from build123d import *

# Parameters (mm, degrees)
SKETCH2_W           = 500
SKETCH2_H           = 500
BOSS_EXTRUDE1_DEPTH = 50
SKETCH7_W           = 400
SKETCH7_H           = 400
CUT_EXTRUDE1_DEPTH  = 550
SKETCH8_W           = 500
SKETCH8_H           = 10
BOSS_EXTRUDE2_DEPTH = 10
SKETCH9_W           = 50
SKETCH9_H           = 50
BOSS_EXTRUDE3_DEPTH = 550
SKETCH10_W          = 50
SKETCH10_H          = 50
BOSS_EXTRUDE4_DEPTH = 600


with BuildPart() as part:
    # Sketch2 → Boss-Extrude1 (new body)
    with BuildSketch(Plane(origin=(0, 0, 0), x_dir=(1, 0, 0), z_dir=(0, 1, 0))):
        Rectangle(SKETCH2_W, SKETCH2_H)
    extrude(amount=BOSS_EXTRUDE1_DEPTH)

    # Sketch7 → Cut-Extrude1 (cut)
    with BuildSketch(Plane(origin=(0, 50, 0), x_dir=(1, 0, 0), z_dir=(0, 1, 0))):
        Rectangle(SKETCH7_W, SKETCH7_H)
    extrude(amount=-CUT_EXTRUDE1_DEPTH, mode=Mode.SUBTRACT)

    # Sketch8 → Boss-Extrude2 (add)
    with BuildSketch(Plane(origin=(0, 50, 0), x_dir=(1, 0, 0), z_dir=(0, 1, 0))):
        with Locations((0, 235)):
            Rectangle(SKETCH8_W, SKETCH8_H)
        with Locations((0, -235)):
            Rectangle(SKETCH8_W, SKETCH8_H)
    extrude(amount=BOSS_EXTRUDE2_DEPTH)

    # Sketch9 → Boss-Extrude3 (add)
    with BuildSketch(Plane.XZ):
        with Locations((125, -275)):
            Rectangle(SKETCH9_W, SKETCH9_H)
        with Locations((125, 275)):
            Rectangle(SKETCH9_W, SKETCH9_H)
    extrude(amount=-BOSS_EXTRUDE3_DEPTH)

    # Sketch10 → Boss-Extrude4 (add)
    with BuildSketch(Plane.XY.offset(300)):
        with Locations((125, 575)):
            Rectangle(SKETCH10_W, SKETCH10_H)
    extrude(amount=-BOSS_EXTRUDE4_DEPTH)


solid = part.part
Check sheet for the modelled part. Datum: model origin and axes. Units: mm. A direction names the side the tool comes from. Give positions to 0.01 mm unless a question says otherwise; leave off trailing zeros. Loops run counter-clockwise (first coordinate to the right, second up) from the corner with the lowest first, then second, coordinate; pieces in that order, holes last. Notation, with made-up numbers: M 45.5,-12 L 65.5,-12 A5 cw 65.5,-6 Z; hole C -20,35 d4. An arc over 180 degrees is marked long. Use a Markdown table: item, result. Add a question column.
Q1. Sectioned sample at C-C, the plane z = 178.5. Record the cut outline in (x, y).
Q2. Sectioned sample at D-D, the plane x = -217.5. Record the cut outline in (y, z), then the cut area to 3 significant figures.
Q3. Scan lines: line 1 along Y through (x, z) = (24, 244); line 2 along X through (y, z) = (430.5, 250.5); line 3 along Z through (x, y) = (-93, 42). Record each from-to range of solid material in increasing order. Write a range as [from, to].
Q4. Sectioned sample at B-B, the plane x = -18. Record the cut outline in (y, z), then the cut area to 3 significant figures.
Q5. Mould release check, pull along Y, two halves, no side actions. Record for faces 1 (the flat face through (125, 296, -250)), 2 (the flat face through (200, 25, 3)), 3 (the flat face through (125, 600, 4)): pulls with the +Y half, pulls with the -Y half, needs draft (parallel to the pull), parting line crosses it, or undercut.
Q6. Tool access check on faces 4 (the flat face through (199, 25, 250)), 5 (the flat face through (-200, 25, 3)), 6 (the flat face through (-77, 25, 250)). Record the directions out of +Z, -Z, +X, -X, +Y, -Y that give a thin tool (end or side, any length) a straight path to the whole face; none if there is none.
Q7. Sectioned sample at A-A, the plane y = 356. Record the cut outline in (x, z), then the cut area to 3 significant figures.
Q8. Go/stop test with flat-tipped pins: pin 1 (25 mm diameter, centred on x = 133.5, z = -35, fed in from -Y); pin 2 (11 mm diameter, centred on x = 46.5, y = 55, fed in from +Z); pin 3 (25 mm diameter, centred on x = -93.5, y = 36, fed in from -Z). Record where each tip stops, or that it passes through.
Verdict:
| question | item | result |
|---|---|---|
| 1 | outline | M -250,0 L -200,0 L -200,50 L -250,50 Z; M 100,550 L 150,550 L 150,600 L 100,600 Z; M 200,0 L 250,0 L 250,50 L 200,50 Z |
| 2 | outline | M 0,-250 L 50,-250 L 50,-240 L 60,-240 L 60,-230 L 50,-230 L 50,230 L 60,230 L 60,240 L 50,240 L 50,250 L 0,250 Z |
| 2 | area | 25,200 mm^2 |
| 3 | line 1 | [0, 50] |
| 3 | line 2 | [100, 150] |
| 3 | line 3 | [-250, -200], [200, 250] |
| 4 | outline | M 0,-250 L 50,-250 L 50,-240 L 60,-240 L 60,-230 L 50,-230 L 50,-200 L 0,-200 Z; M 0,200 L 50,200 L 50,230 L 60,230 L 60,240 L 50,240 L 50,250 L 0,250 Z |
| 4 | area | 5,200 mm^2 |
| 5 | face 1 | undercut |
| 5 | face 2 | needs draft |
| 5 | face 3 | pulls with the +Y half |
| 6 | face 4 | +Z, +X, +Y, -Y |
| 6 | face 5 | +Y, -Y |
| 6 | face 6 | +Z, -X, +Y, -Y |
| 7 | outline | M 100,-300 L 150,-300 L 150,-250 L 100,-250 Z; M 100,250 L 150,250 L 150,300 L 100,300 Z |
| 7 | area | 5,000 mm^2 |
| 8 | pin 1 | y = 550 |
| 8 | pin 2 | z = 250 |
| 8 | pin 3 | z = -250 |
